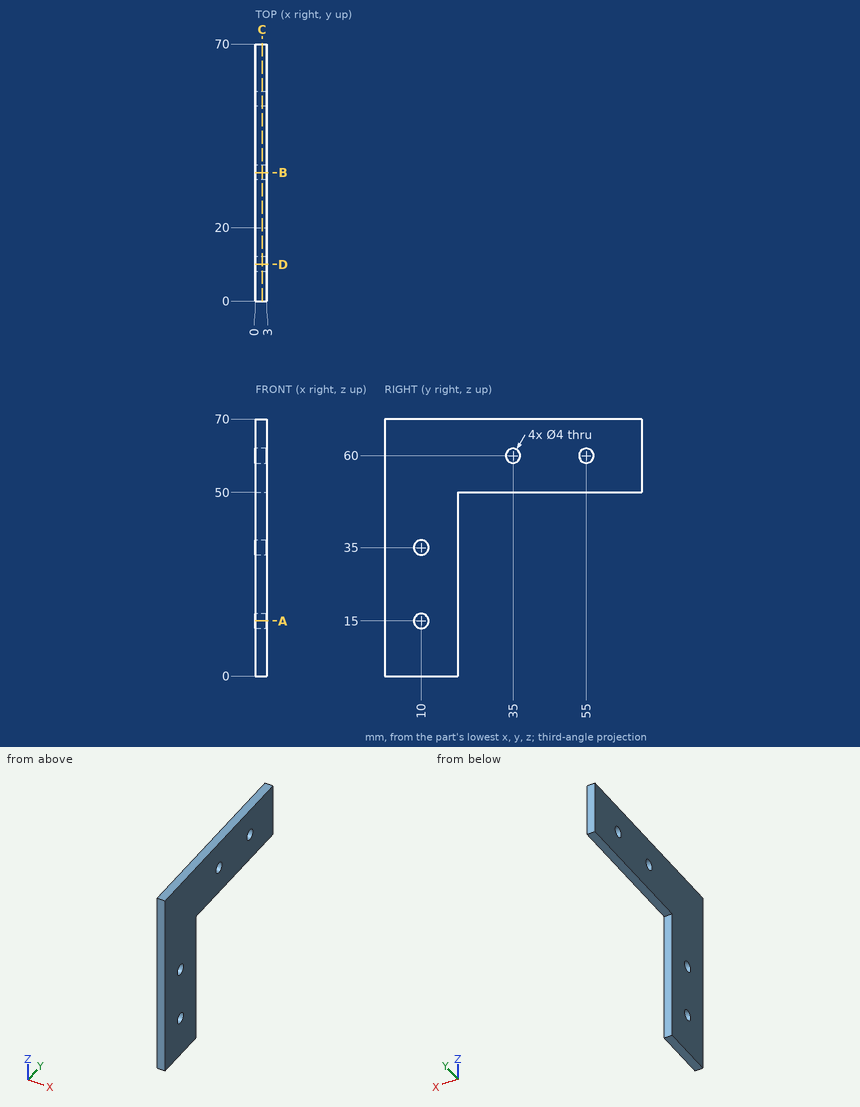
Print and shaded views of the part. All mm, measured from the part's lowest x, y and z. Coordinates: 2 decimals unless noted, no trailing zeros. Write each loop counter-clockwise with the first axis right and the second up, starting at its lowest first coordinate (ties: lowest second). Pieces come first, ordered by that corner, then holes. Notation, with made-up numbers: M 31.25,53.25 L 50.25,53.25 A11 cw 50.25,63.25 Z; hole C -27.75,14 d6. An arc over 180 degrees is marked long. Return JSON: item names as keys, results as strings.
1. Flat gauge pin, fed straight in: pin 1 Ø1.5 at (x, y) = (2, 55.5) entering from -Z. Where does the tip first touch, or does it go through?
Determined:
{"pin 1": "z = 50"}
2. Probe L1, parallel to Y at x = 2.2, z = 60; L2, parallel to Y at x = 2.35, z = 35; L3, parallel to Z at x = 0.3, y = 29. List the from-to ranges inside material, lowest first.
Determined:
{"L1": "0 to 33, 37 to 53, 57 to 70", "L2": "0 to 8, 12 to 20", "L3": "50 to 70"}
3. Saw through at B-B, the plane y = 35. Write the cut outline in (x, z), then the cut area to 3 significant figures.
Determined:
{"outline": "M 0,50 L 3,50 L 3,58 L 0,58 Z; M 0,62 L 3,62 L 3,70 L 0,70 Z", "area": "48.0 mm²"}
4. Saw through at C-C, the plane x = 1.8. Write the cut outline in (y, z), then the cut area to 3 significant figures.
Determined:
{"outline": "M 0,0 L 20,0 L 20,50 L 70,50 L 70,70 L 0,70 Z; hole C 10,15 d4; hole C 10,35 d4; hole C 35,60 d4; hole C 55,60 d4", "area": "2,350 mm²"}
5. Saw through at A-A, the plane z = 15. Write the cut outline in (x, y).
Determined:
{"outline": "M 0,0 L 3,0 L 3,8 L 0,8 Z; M 0,12 L 3,12 L 3,20 L 0,20 Z"}
6. Saw through at D-D, the plane y = 10. Write the cut outline in (x, z).
Determined:
{"outline": "M 0,0 L 3,0 L 3,13 L 0,13 Z; M 0,17 L 3,17 L 3,33 L 0,33 Z; M 0,37 L 3,37 L 3,70 L 0,70 Z"}
